Check sheet for the modelled part. Datum: model origin and axes. Units: mm. A direction names the side the tool comes from. Give positions to 0.01 mm unless a question says otherwise; leave off trailing zeros. Write each loop counter-clockwise with the first axis right and the second up, starting at its lowest first coordinate (ties: lowest second). Pieces come first, ordered by that corner, then holes. Notation, with made-up numbers: (51.25, 38.25) -> (75.25, 38.25) arc R25 ccw to (75.25, 61.25) -> close; hole circle Ø1 at (82, 17). An arc over 180 degrees is marked (long way). Answer as a JSON object with one key per item and string values.
from build123d import *
from build123d.topology import SkipClean

# Parameters (mm, degrees)
BOSS_EXTRUDE2_DEPTH = 1
SKETCH2_R           = 2.5
SKETCH2_R_2         = 1.159513831
BOSS_EXTRUDE3_DEPTH = 1.5


with BuildPart() as part:
    # Sketch1 → Boss-Extrude2 (new, symmetric)
    with BuildSketch(Plane.XY):
        with BuildLine():
            ThreePointArc((-12.5, 0), (-13.232233047, -1.767766953), (-15, -2.5))
            Line((-15, -2.5), (0, -2.5))
            ThreePointArc((0, -2.5), (-2.5, -1.2e-08), (-2.3e-08, 2.5))
            Line((-2.3e-08, 2.5), (-15, 2.5))
            ThreePointArc((-15, 2.5), (-13.232233047, 1.767766953), (-12.5, 0))
        make_face()
        with BuildLine():
            ThreePointArc((-15, 2.5), (-17.5, 0), (-15, -2.5))
            Line((-15, -2.5), (-15, -0.25))
            ThreePointArc((-15, -0.25), (-15.25, 0), (-15, 0.25))
            Line((-15, 0.25), (-15, 2.5))
        make_face()
        with BuildLine():
            Line((-15, -0.25), (-15, -2.5))
            ThreePointArc((-15, -2.5), (-13.232233047, -1.767766953), (-12.5, 0))
            ThreePointArc((-12.5, 0), (-13.232233047, 1.767766953), (-15, 2.5))
            Line((-15, 2.5), (-15, 0.25))
            ThreePointArc((-15, 0.25), (-14.823223305, 0.176776695), (-14.75, 0))
            ThreePointArc((-14.75, 0), (-14.823223305, -0.176776695), (-15, -0.25))
        make_face()
        with BuildLine():
            ThreePointArc((-15, 2.5), (-17.5, 0), (-15, -2.5))
            Line((-15, -2.5), (-15, -0.25))
            ThreePointArc((-15, -0.25), (-15.25, 0), (-15, 0.25))
            Line((-15, 0.25), (-15, 2.5))
        make_face()
        with BuildLine():
            Line((-15, -0.25), (-15, -2.5))
            ThreePointArc((-15, -2.5), (-13.232233047, -1.767766953), (-12.5, 0))
            ThreePointArc((-12.5, 0), (-13.232233047, 1.767766953), (-15, 2.5))
            Line((-15, 2.5), (-15, 0.25))
            ThreePointArc((-15, 0.25), (-14.823223305, 0.176776695), (-14.75, 0))
            ThreePointArc((-14.75, 0), (-14.823223305, -0.176776695), (-15, -0.25))
        make_face()
        with BuildLine():
            ThreePointArc((2.5, 0), (1.767766953, -1.767766953), (0, -2.5))
            Line((0, -2.5), (15, -2.5))
            ThreePointArc((15, -2.5), (12.5, 0), (15, 2.5))
            Line((15, 2.5), (-2.3e-08, 2.5))
            ThreePointArc((-2.3e-08, 2.5), (1.767766945, 1.767766961), (2.5, 0))
        make_face()
        with BuildLine():
            ThreePointArc((15, 2.5), (12.5, 0), (15, -2.5))
            Line((15, -2.5), (15, -0.25))
            ThreePointArc((15, -0.25), (14.75, 0), (15, 0.25))
            Line((15, 0.25), (15, 2.5))
        make_face()
        with BuildLine():
            Line((15, -0.25), (15, -2.5))
            ThreePointArc((15, -2.5), (16.767766953, -1.767766953), (17.5, 0))
            ThreePointArc((17.5, 0), (16.767766953, 1.767766953), (15, 2.5))
            Line((15, 2.5), (15, 0.25))
            ThreePointArc((15, 0.25), (15.176776695, 0.176776695), (15.25, 0))
            ThreePointArc((15.25, 0), (15.176776695, -0.176776695), (15, -0.25))
        make_face()
        with BuildLine():
            ThreePointArc((15, 2.5), (12.5, 0), (15, -2.5))
            Line((15, -2.5), (15, -0.25))
            ThreePointArc((15, -0.25), (14.75, 0), (15, 0.25))
            Line((15, 0.25), (15, 2.5))
        make_face()
        with BuildLine():
            Line((15, -0.25), (15, -2.5))
            ThreePointArc((15, -2.5), (16.767766953, -1.767766953), (17.5, 0))
            ThreePointArc((17.5, 0), (16.767766953, 1.767766953), (15, 2.5))
            Line((15, 2.5), (15, 0.25))
            ThreePointArc((15, 0.25), (15.176776695, 0.176776695), (15.25, 0))
            ThreePointArc((15.25, 0), (15.176776695, -0.176776695), (15, -0.25))
        make_face()
    extrude(amount=BOSS_EXTRUDE2_DEPTH, both=True)

    # Sketch2 → Boss-Extrude3 (add, symmetric)
    with SkipClean():  # the faces are left unmerged after this step: merging them gives an invalid solid
        with BuildSketch(Plane.XY):
            with Locations(Location((0, 0, 0), (0, 0, 270))):
                Circle(SKETCH2_R)
            Circle(SKETCH2_R_2, mode=Mode.SUBTRACT)
        extrude(amount=BOSS_EXTRUDE3_DEPTH, both=True)


solid = part.part
1. Sectioned sample at C-C, the plane x = -14. Enter the section's corners in (y, z).
Determined:
{"outline": "(-2.5, -1) -> (2.5, -1) -> (2.5, 1) -> (-2.5, 1) -> close"}
2. Sectioned sample at A-A, the plane z = 0.4. Enter the section's corners in (x, y), plus the area to 3 significant figures.
Determined:
{"outline": "(-15, -2.5) -> (15, -2.5) arc R2.5 ccw to (15, 2.5) -> (-15, 2.5) arc R2.5 ccw to start; hole circle Ø0.5 at (-15, 0); hole circle Ø2.32 at (0, 0); hole circle Ø0.5 at (15, 0)", "area": "165 mm^2"}
3. Go/stop test with flat-tipped pins: P1, Ø1.5, axis at x = -9.5, y = -1, coming from the +Z side; P2, Ø2.5, axis at x = -9.5, y = -1, coming from the -Z side. Record where each tip stops, or that it passes through.
Determined:
{"P1": "z = 1", "P2": "z = -1"}
4. Access from +Z, -Z, +X, -X, +Y, -Y to the whole of each face (thin tool, end or side, straight path). Record for faces 1 (the face through (-0.96, -2.31, -1.25)), 2 (the face through (-0.96, -2.31, 1.25)), 3 (the face through (-1, -1, 1.5)).
Determined:
{"face 1": "-Z", "face 2": "+Z", "face 3": "+Z, +X, -X, +Y, -Y"}
5. Scan lines: L1, parallel to Y at x = 0, z = 1; L2, parallel to Z at x = -6.5, y = -1.05; L3, parallel to X at y = 0.1, z = -0.5. Record each from-to range of solid material in increasing order. Write a range as [from, to].
Determined:
{"L1": "[-2.5, -1.16], [1.16, 2.5]", "L2": "[-1, 1]", "L3": "[-17.5, -15.23], [-14.77, -1.16], [1.16, 14.77], [15.23, 17.5]"}
6. Sectioned sample at B-B, the plane x = 1.5. Enter the section's corners in (y, z).
Determined:
{"outline": "(-2.5, -1) -> (-2, -1) -> (-2, -1.5) -> (2, -1.5) -> (2, -1) -> (2.5, -1) -> (2.5, 1) -> (2, 1) -> (2, 1.5) -> (-2, 1.5) -> (-2, 1) -> (-2.5, 1) -> close"}
